Check sheet for the drawn part. Datum: minimum x, y, z corner. Units: mm. A direction names the side the tool comes from. Round coordinates to 2 decimals unless told otherwise and drop trailing zeros. Write each loop counter-clockwise with the first axis right and the second up, starting at its lowest first coordinate (ties: lowest second). Pieces come first, ordered by that corner, then holes. Notation, with made-up numbers: M 45,-20 L 103,-20 A14 ccw 103,0 Z; hole C -3.5,23 d5. An arc over 180 degrees is marked long. Put each result on its own line as item: value.
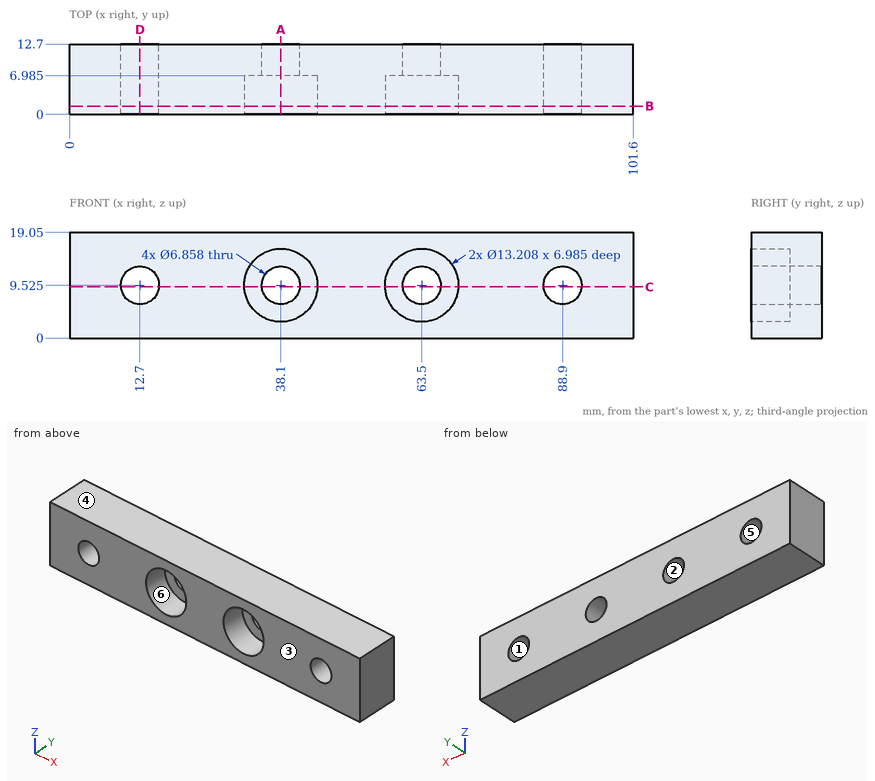
1. Cross-section at B-B (y = 1.5). Enter the section's corners in (x, z) (3 decimals).
Computed values:
outline: M 0,0 L 101.6,0 L 101.6,19.05 L 0,19.05 Z; hole C 12.7,9.525 d6.858; hole C 38.1,9.525 d13.208; hole C 63.5,9.525 d13.208; hole C 88.9,9.525 d6.858
2. Release check for a two-part mould opening along Z. For the marked faces 1, 2, 3 and 4 record: +Z half, -Z half, draft (parallel to the pull), parting line (faces both ways), or undercut.
Computed values:
face 1: undercut
face 2: undercut
face 3: draft
face 4: +Z half
3. Cross-section at A-A (x = 38.1). Enter the section's corners in (y, z) (3 decimals), then the cut area to 3 significant figures.
Computed values:
outline: M 0,0 L 12.7,0 L 12.7,6.096 L 6.985,6.096 L 6.985,2.921 L 0,2.921 Z; M 0,16.129 L 6.985,16.129 L 6.985,12.954 L 12.7,12.954 L 12.7,19.05 L 0,19.05 Z
area: 110 mm2
4. Cross-section at D-D (x = 12.7). Enter the section's corners in (y, z), then the cut area to 3 significant figures.
Computed values:
outline: M 0,0 L 12.7,0 L 12.7,6.1 L 0,6.1 Z; M 0,12.95 L 12.7,12.95 L 12.7,19.05 L 0,19.05 Z
area: 155 mm2
5. Scan lines: probe 1 along X at (y, z) = (4, 9.25); probe 2 along Z at (x, y) = (40.5, 10); probe 3 along X at (y, z) = (4, 13.75). Record each from-to range of solid material in increasing order.
Computed values:
probe 1: x = 0 to 9.28, 16.12 to 31.5, 44.7 to 56.9, 70.1 to 85.48, 92.32 to 101.6
probe 2: z = 0 to 7.08, 11.97 to 19.05
probe 3: x = 0 to 33.02, 43.18 to 58.42, 68.58 to 101.6
6. Depth check by flat-ended pin: pin 1 Ø11 at (x, z) = (63.5, 9.525) entering from -Y (3 decimals); pin 2 Ø5.5 at (x, z) = (88.9, 9.525) entering from +Y (1 decimal). Enter the tip coordinate at first touch or a pass-through.
Computed values:
pin 1: stops at y = 6.985
pin 2: passes through
7. Cross-section at C-C (z = 9.25). Enter the section's corners in (x, y) (3 decimals), then the cut area to 3 significant figures.
Computed values:
outline: M 0,0 L 9.282,0 L 9.282,12.7 L 0,12.7 Z; M 16.118,0 L 31.502,0 L 31.502,6.985 L 34.682,6.985 L 34.682,12.7 L 16.118,12.7 Z; M 41.518,6.985 L 44.698,6.985 L 44.698,0 L 56.902,0 L 56.902,6.985 L 60.082,6.985 L 60.082,12.7 L 41.518,12.7 Z; M 66.918,6.985 L 70.098,6.985 L 70.098,0 L 85.482,0 L 85.482,12.7 L 66.918,12.7 Z; M 92.318,0 L 101.6,0 L 101.6,12.7 L 92.318,12.7 Z
area: 854 mm2
8. Access from +Z, -Z, +X, -X, +Y, -Y to the whole of each face (thin tool, end or side, straight path). Record for the marked faces 5 and 6.
Computed values:
face 5: +Y, -Y
face 6: -Y
